The model under review builds one solid part; all positions refer to its coordinate system, in mm. A direction names the side the tool comes from. Round coordinates to 2 decimals unless told otherwise and drop trailing zeros. Loops run counter-clockwise (first coordinate to the right, second up) from the corner with the lowest first, then second, coordinate; pieces in that order, holes last. Notation, with made-up numbers: (84.5, -10) - (88.5, -10) arc R27 ccw to (88.5, 13) - close; hole circle Ø7 at (24, -32.5). An arc over 180 degrees is marked (long way). Answer as CSV lines item,"result".
from build123d import *

# Parameters (mm, degrees)
F0_R     = 2.2479
F1_DEPTH = 3.048
F0_W     = 50.8
F0_H     = 3.1029520094
F0_W_2   = 3.3275114092
F0_H_2   = 44.704
F0_W_3   = 2.7684885908
F2_DEPTH = 25.4
F4_R     = 2.54
F6_DEPTH = 25.4
F7_DEPTH = 25.4


with BuildPart() as f1:
    # F0 (on Front) → F1 (new body)
    with BuildSketch(Plane.XZ):
        Polygon((30.5415683826, 28.2853763875), (-26.3544316174, 28.2853763875), (-26.3544316174, -16.4186236125), (-23.0269202082, -16.4186236125), (-23.0269202082, -19.5215756219), (27.7730797918, -19.5215756219), (27.7730797918, -16.4186236125), (30.5415683826, -16.4186236125), align=None)
        with Locations((-10.7998287971, 18.1253763875)):
            Circle(F0_R, mode=Mode.SUBTRACT)
        with Locations((14.6001712029, 18.1253763875)):
            Circle(F0_R, mode=Mode.SUBTRACT)
    extrude(amount=F1_DEPTH)

    # F0 (on Front) → F2 (join)
    with BuildSketch(Plane.XZ):
        with Locations((2.3730797918, -21.0730516266)):
            Rectangle(F0_W, F0_H)
        with Locations((-28.018187322, 5.9333763875)):
            Rectangle(F0_W_2, F0_H_2)
        with Locations((31.925812678, 5.9333763875)):
            Rectangle(F0_W_3, F0_H_2)
    extrude(amount=F2_DEPTH)

    # F4
    f4_edges = [f1.edges().sort_by_distance(p)[0] for p in [
        (2.37308, -3.048, -19.521576),
        (2.37308, 0, -22.624528),
        (33.310057, 0, 5.933376),
        (30.541568, -3.048, 5.933376),
        (-26.354432, -3.048, 5.933376),
        (-29.681943, 0, 5.933376),
    ]]
    fillet(f4_edges, radius=F4_R)

    # F5 (on face) → F6 (cut)
    with BuildSketch(Plane(origin=(30.5415683826, 0, 0), x_dir=(0, -1, 0), z_dir=(-1, 0, 0))):
        with BuildLine():
            ThreePointArc((20.1026303179, 20.6653763875), (16.6749283671, 24.0930783383), (13.2472264163, 20.6653763875))
            Line((13.2472264163, 20.6653763875), (13.2472264163, -8.7986236125))
            ThreePointArc((13.2472264163, -8.7986236125), (16.6749283671, -12.2263255633), (20.1026303179, -8.7986236125))
            Line((20.1026303179, -8.7986236125), (20.1026303179, 20.6653763875))
        make_face()
    extrude(amount=-F6_DEPTH, mode=Mode.SUBTRACT)

    # F3 (on face) → F7 (cut)
    with BuildSketch(Plane.XY.offset(-19.5215756219)):
        with BuildLine():
            ThreePointArc((-15.1830099327, -12.3297252466), (-17.7230099327, -14.8697252466), (-15.1830099327, -17.4097252466))
            Line((-15.1830099327, -17.4097252466), (20.3769900673, -17.4097252466))
            ThreePointArc((20.3769900673, -17.4097252466), (22.9169900673, -14.8697252466), (20.3769900673, -12.3297252466))
            Line((20.3769900673, -12.3297252466), (-15.1830099327, -12.3297252466))
        make_face()
    extrude(amount=-F7_DEPTH, mode=Mode.SUBTRACT)


solid = f1.part
1. Take a section at A-A (z = 2.5). State the section outline as (x, y) points.
Numbers:
outline,"(-29.68, -25.4) - (-26.35, -25.4) - (-26.35, -5.59) arc R2.54 cw to (-23.81, -3.05) - (28, -3.05) arc R2.54 cw to (30.54, -5.59) - (30.54, -13.25) - (33.31, -13.25) - (33.31, -2.54) arc R2.54 ccw to (30.77, 0) - (-27.14, 0) arc R2.54 ccw to (-29.68, -2.54) - close; (30.54, -25.4) - (33.31, -25.4) - (33.31, -20.1) - (30.54, -20.1) - close"
2. Clearance check with flat-ended pins moving along their axes: pin 1 (7 mm diameter, centred on y = -7, z = -20.5, fed in from +X); pin 2 (3 mm diameter, centred on x = -21.5, y = -15.5, fed in from +Z); pin 3 (7 mm diameter, centred on x = 14.6, z = 18.13, fed in from -Y). State where each tip first meets the part, or that it passes through.
Numbers:
pin 1,"stops at x = 27.77"
pin 2,"stops at z = -19.52"
pin 3,"stops at y = -3.05"
3. Take a section at C-C (x = 3). State the section outline as (y, z) points.
Numbers:
outline,"(-25.4, -22.62) - (-17.41, -22.62) - (-17.41, -19.52) - (-25.4, -19.52) - close; (-12.33, -22.62) - (-2.54, -22.62) arc R2.54 ccw to (0, -20.08) - (0, 28.29) - (-3.05, 28.29) - (-3.05, -16.98) arc R2.54 cw to (-5.59, -19.52) - (-12.33, -19.52) - close"
4. Wall thickness on probe 1 along X at (y, z) = (-14, -15); probe 2 along Z at (x, y) = (0, -6); probe 3 along Y at (x, z) = (2.5, -14): over which ranges is each line inside the solid? List them lowest first.
Numbers:
probe 1,"x = -29.68 to -26.35, 30.54 to 33.31"
probe 2,"z = -22.62 to -19.52"
probe 3,"y = -3.05 to 0"
5. Take a section at D-D (y = -14.5). State the section outline as (x, z) points, plus the area to 3 significant figures.
Numbers:
outline,"(-29.68, -16.42) - (-26.35, -16.42) - (-26.35, 28.29) - (-29.68, 28.29) - close; (-23.03, -22.62) - (-17.7, -22.62) - (-17.7, -19.52) - (-23.03, -19.52) - close; (22.89, -22.62) - (27.77, -22.62) - (27.77, -19.52) - (22.89, -19.52) - close; (30.54, -16.42) - (33.31, -16.42) - (33.31, -11.45) - (30.54, -11.45) - close; (30.54, 23.31) - (33.31, 23.31) - (33.31, 28.29) - (30.54, 28.29) - close"
area,"208 mm²"
6. Draft analysis for pull direction X (two halves, no side actions). For faces 4 (the face through (-17.722, -14.814, -21.051)), 5 (the face through (-23.027, -13, -21)), 6 (the face through (33.31, -11, 6)), 7 (the face through (32, -25.4, 6)), state which applies: +X half, -X half, draft (parallel to the pull), parting line (faces both ways), or undercut.
Numbers:
face 4,"undercut"
face 5,"-X half"
face 6,"+X half"
face 7,"draft"
7. Tool access review of faces 1 (the face through (32, -20.103, 6)), 2 (the face through (22.916, -14.926, -21.051)), 3 (the face through (-28, -13, -16.419)): name each direction out of +Z, -Z, +X, -X, +Y, -Y from which nothing blocks a thin tool from reaching the whole face with its end or side.
Numbers:
face 1,"+X"
face 2,"+Z, -Z"
face 3,"-Z, -X, +Y, -Y"
8. Take a section at B-B (y = -9.5). State the section outline as (x, z) points.
Numbers:
outline,"(-29.68, -16.42) - (-26.35, -16.42) - (-26.35, 28.29) - (-29.68, 28.29) - close; (-23.03, -22.62) - (27.77, -22.62) - (27.77, -19.52) - (-23.03, -19.52) - close; (30.54, -16.42) - (33.31, -16.42) - (33.31, 28.29) - (30.54, 28.29) - close"
